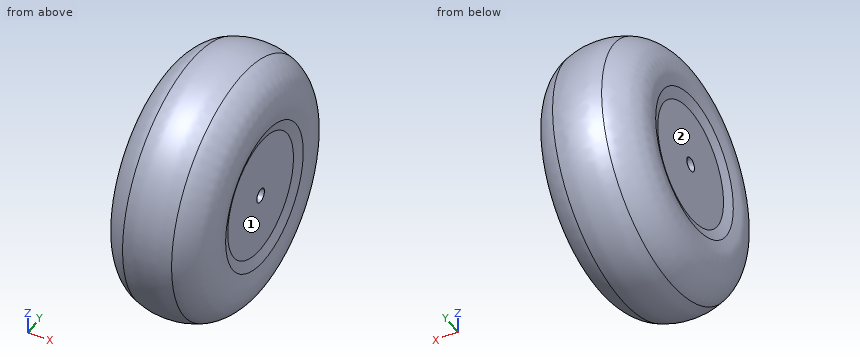
```python
from build123d import *

# Parameters (mm, degrees)
SKETCH1_R               = 17.25
BOSS_EXTRUDE1_DEPTH     = 26
FILLET1_R               = 20
FILLET2_R               = 12
SKETCH3_R               = 2
CUT_EXTRUDE1_DEPTH      = 2.795288953
CUT_EXTRUDE1_DEPTH_BACK = 28.795288953


with BuildPart() as part:
    # Sketch1 → Boss-Extrude1 (new body)
    with BuildSketch(Plane(origin=(0, 0, 0), x_dir=(0, 0, -1), z_dir=(1, 0, 0))):
        Circle(SKETCH1_R)
    extrude(amount=BOSS_EXTRUDE1_DEPTH)

    # Sketch2 → Revolve1 (revolve)
    with BuildSketch(Plane.XY):
        with BuildLine():
            Line((-4.622703996, 30.25), (0, 17.25))
            Line((0, 17.25), (26, 17.25))
            Line((26, 17.25), (30.622703996, 30.25))
            ThreePointArc((30.622703996, 30.25), (22.131370856, 34.751946348), (13, 37.75))
            ThreePointArc((13, 37.75), (3.868629144, 34.751946348), (-4.622703996, 30.25))
        make_face()
    revolve(axis=Axis((0, 0, 0), (1, 0, 0)))

    # Fillet1
    fillet1_edges = [part.edges().sort_by_distance(p)[0] for p in [
        (13, -37.75, 0),
    ]]
    fillet(fillet1_edges, radius=FILLET1_R)

    # Fillet2
    fillet2_edges = [part.edges().sort_by_distance(p)[0] for p in [
        (-4.622703996, -30.25, 0),
        (30.622703996, -30.25, 0),
    ]]
    fillet(fillet2_edges, radius=FILLET2_R)

    # Sketch3 → Cut-Extrude1 (cut, two sides)
    with BuildSketch(Plane.ZY) as cut_extrude1_sk:
        Circle(SKETCH3_R)
    extrude(amount=CUT_EXTRUDE1_DEPTH, mode=Mode.SUBTRACT)
    extrude(cut_extrude1_sk.sketch, amount=-CUT_EXTRUDE1_DEPTH_BACK, mode=Mode.SUBTRACT)


solid = part.part
```
Here's how the part is built. I have some questions about the finished solid (model axes, mm). Face numbers are marked on the shaded views. A direction names the side the tool comes from. Give positions to 0.01 mm unless a question says otherwise; leave off trailing zeros. Use one line per item in the form item = value. Start each with the question number.
1) For P1, Ø8, axis at x = 8.5, y = 18, coming from the +Z side; P2, Ø10.5, axis at y = 1.5, z = -4, coming from the +X side; P3, Ø1, axis at y = 28.5, z = 0, coming from the -X side; P4, Ø3.5, axis at y = 0, z = 0, coming from the -X side, each with a flat end and sliding along its axis, tell me the tip position at first contact or that it passes through.
2) Please list where these lines run through material, in increasing order: line 1 along X through (y, z) = (3, 12); line 2 along X through (y, z) = (-22.5, 10); line 3 along Y through (x, z) = (11, 3.5).
3) Which directions (+Z, -Z, +X, -X, +Y, -Y) give clear straight access to the entire face, cutting with the end or side of a thin tool? Please do the marked faces 1 and 2.
Check values:
q1.P1 = 33.75
q1.P2 = 26
q1.P3 = -1.23
q1.P4 = through
q2.line_1 = 0 to 26
q2.line_2 = -1.79 to 27.79
q2.line_3 = -36.61 to 36.61
q3.face_1 = +X
q3.face_2 = -X
